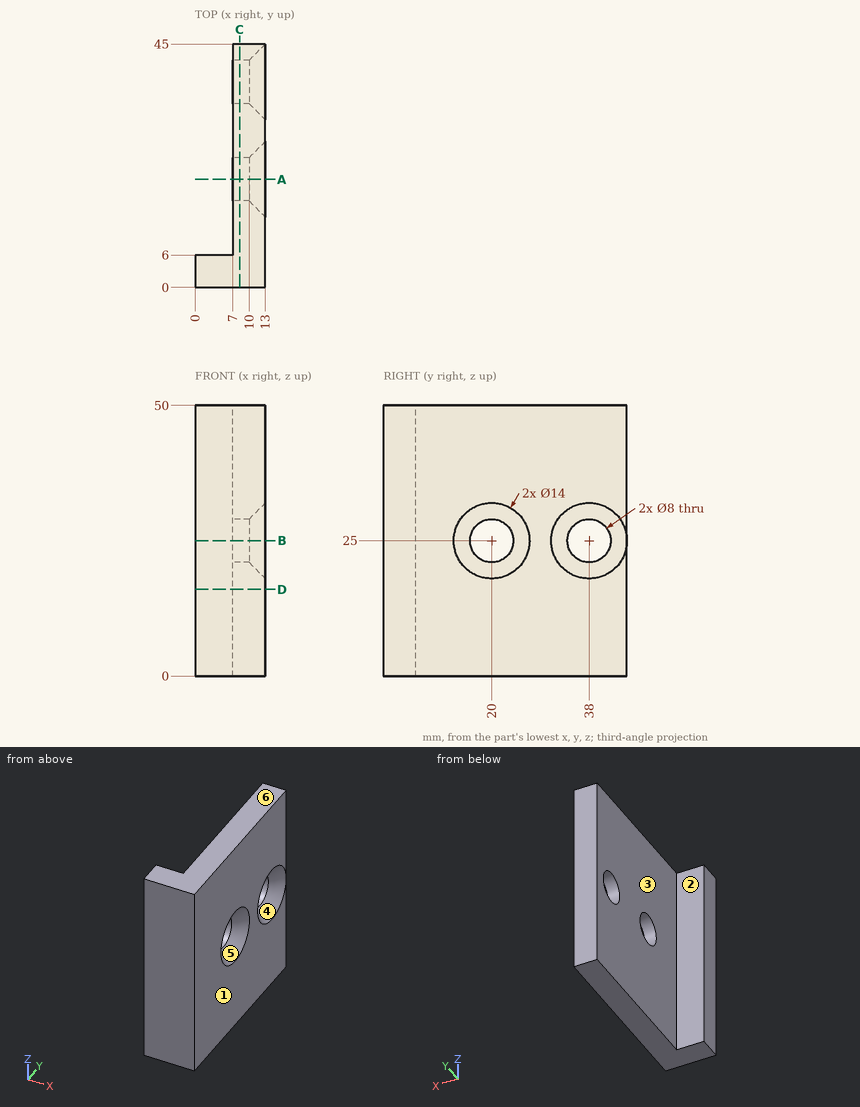
Answer from the drawing. Dimensions are ordinates in mm from the lowest x, y and z of the part. A direction names the side the tool comes from. Give positions to 0.01 mm unless a question says otherwise; leave off trailing zeros. Write each loop counter-clockwise with the first axis right and the second up, starting at its lowest first coordinate (ties: lowest second). Pieces come first, ordered by that corner, then holes. Notation, with made-up numbers: (67, 45.25) - (120, 45.25) arc R30 cw to (120, 74.25) - close; hole circle Ø7 at (43, 43). An arc over 180 degrees is marked (long way). One line per item, written item: value. Start each with the question number.
1. Find section B-B (z = 25). State how many separate pieces and enclosed holes the cut face has, then the cut area to 3 significant figures.
2. For the marked faces 1 and 2, determine the directions among +Z, -Z, +X, -X, +Y, -Y from which every point of the face is accessible in a straight line to the end or side of a thin tool.
3. Given pin 1 (5 mm diameter, centred on y = 38, z = 25, fed in from -X); pin 2 (3 mm diameter, centred on x = 6.5, z = 20, fed in from +Y); pin 3 (3.5 mm diameter, centred on x = 4, z = 36.5, fed in from +Y); pin 4 (4 mm diameter, centred on y = 19.5, z = 27, fed in from +X), each flat-ended and moving along its own axis, determine where each tip first touches the part or whether it passes through.
4. Find section C-C (x = 8.25). Write down the section's boundary in (y, z), then the cut area to 3 significant figures.
5. For a pull along Z with two mould halves and no side action, classify the marked faces 3, 4, 5 and 6 as +Z half, -Z half, draft (parallel to the pull), parting line (faces both ways), or undercut.
6. Consider probe 1 along Y at (x, z) = (7.8, 25); probe 2 along Y at (x, z) = (11, 23.5); probe 3 along X at (y, z) = (8.5, 34). Determine where each line is inside the solid, lowest interval first.
7. Find section A-A (y = 20). Write down the section's boundary in (x, z).
8. Find section D-D (z = 16). Write down the section's boundary in (x, y).
Geometry results:
1. separate pieces: 3
1. enclosed holes: 0
1. area: 198 mm2
2. face 1: +Z, -Z, +X, +Y, -Y
2. face 2: +Z, -Z, -X, +Y
3. pin 1: through
3. pin 2: y = 45
3. pin 3: y = 6
3. pin 4: x = 10.06
4. outline: (0, 0) - (45, 0) - (45, 50) - (0, 50) - close; hole circle Ø8 at (20, 25); hole circle Ø8 at (38, 25)
4. area: 2,150 mm2
5. face 3: draft
5. face 4: undercut
5. face 5: undercut
5. face 6: +Z half
6. probe 1: 0 to 16, 24 to 34, 42 to 45
6. probe 2: 0 to 15.23, 24.77 to 33.23, 42.77 to 45
6. probe 3: 7 to 13
7. outline: (7, 0) - (13, 0) - (13, 18) - (10, 21) - (7, 21) - close; (7, 29) - (10, 29) - (13, 32) - (13, 50) - (7, 50) - close
8. outline: (0, 0) - (13, 0) - (13, 45) - (7, 45) - (7, 6) - (0, 6) - close
